Work out the finished part from the listing and answer in its coordinate system (mm). Face numbers are marked on the shaded views. Coordinates: 2 decimals unless noted, no trailing zeros. Loops run counter-clockwise (first coordinate to the right, second up) from the corner with the lowest first, then second, coordinate; pieces in that order, holes last. Notation, with made-up numbers: M -10.5,25 L 38.5,25 A22 cw 38.5,31 Z; hole C -15.5,34.25 d4. An arc over 180 degrees is marked long. Write each question's results on one line, items separated by ' | '.
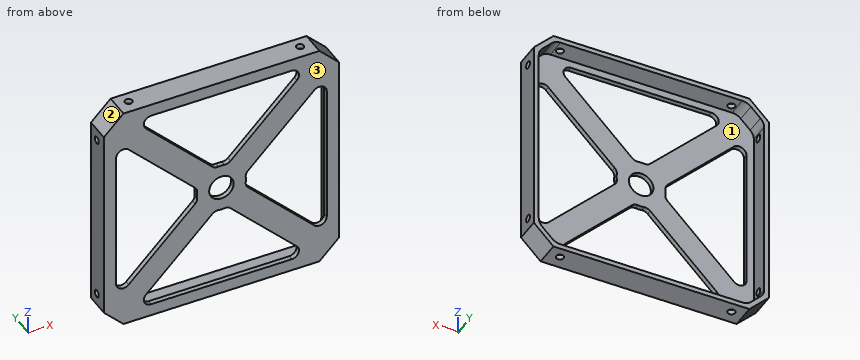
```python
from build123d import *

# Parameters (mm, degrees)
BOSS_EXTRUDE1_DEPTH = 10
SHELL1_T            = -2
SKETCH2_R           = 5
CUT_EXTRUDE1_DEPTH  = 11
FILLET1_R           = 3
SKETCH3_R           = 1.5
CUT_EXTRUDE2_DEPTH  = 97
SKETCH4_R           = 1.5
CUT_EXTRUDE3_DEPTH  = 97
FILLET2_R           = 5


with BuildPart() as part:
    # Sketch1 → Boss-Extrude1 (new body)
    with BuildSketch(Plane(origin=(0, 0, 0), x_dir=(1, 0, 0), z_dir=(0, 1, 0))):
        Polygon((0, 88), (0, 8), (8, 0), (88, 0), (96, 8), (96, 88), (88, 96), (8, 96), align=None)
    extrude(amount=BOSS_EXTRUDE1_DEPTH)

    # Shell1
    shell1_openings = [part.faces().sort_by_distance(p)[0] for p in [
        (48, 10, -48),
    ]]
    offset(amount=SHELL1_T, openings=shell1_openings, kind=Kind.INTERSECTION)

    # Sketch2 → Cut-Extrude1 (cut, through all)
    with BuildSketch(Plane(origin=(0, 0, 0), x_dir=(-1, 0, 0), z_dir=(0, -1, 0))):
        with BuildLine():
            Line((-45.411809549, 57.659258263), (-12.071067812, 91))
            Line((-12.071067812, 91), (-83.928932188, 91))
            Line((-83.928932188, 91), (-50.588190451, 57.659258263))
            ThreePointArc((-50.588190451, 57.659258263), (-48, 58), (-45.411809549, 57.659258263))
        make_face()
        with BuildLine():
            Line((-5, 83.928932188), (-38.340741737, 50.588190451))
            ThreePointArc((-38.340741737, 50.588190451), (-38.085551386, 49.305261922), (-38, 48))
            ThreePointArc((-38, 48), (-38.085551386, 46.694738078), (-38.340741737, 45.411809549))
            Line((-38.340741737, 45.411809549), (-5, 12.071067812))
            Line((-5, 12.071067812), (-5, 83.928932188))
        make_face()
        with BuildLine():
            Line((-12.071067812, 5), (-45.411809549, 38.340741737))
            ThreePointArc((-45.411809549, 38.340741737), (-48, 38), (-50.588190451, 38.340741737))
            Line((-50.588190451, 38.340741737), (-83.928932188, 5))
            Line((-83.928932188, 5), (-12.071067812, 5))
        make_face()
        with BuildLine():
            ThreePointArc((-57.659258263, 45.411809549), (-58, 48), (-57.659258263, 50.588190451))
            Line((-57.659258263, 50.588190451), (-91, 83.928932188))
            Line((-91, 83.928932188), (-91, 12.071067812))
            Line((-91, 12.071067812), (-57.659258263, 45.411809549))
        make_face()
        with Locations((-48, 48)):
            Circle(SKETCH2_R)
    extrude(amount=-CUT_EXTRUDE1_DEPTH, mode=Mode.SUBTRACT)

    # Fillet1
    fillet1_edges = [part.edges().sort_by_distance(p)[0] for p in [
        (50.588190451, 1, -38.340741737),
        (45.411809549, 1, -38.340741737),
        (12.071067812, 1, -5),
        (83.928932188, 1, -5),
        (38.340741737, 1, -45.411809549),
        (38.340741737, 1, -50.588190451),
        (5, 1, -83.928932188),
        (5, 1, -12.071067812),
        (57.659258263, 1, -50.588190451),
        (57.659258263, 1, -45.411809549),
        (91, 1, -12.071067812),
        (91, 1, -83.928932188),
        (45.411809549, 1, -57.659258263),
        (50.588190451, 1, -57.659258263),
        (83.928932188, 1, -91),
        (12.071067812, 1, -91),
    ]]
    fillet(fillet1_edges, radius=FILLET1_R)

    # Sketch3 → Cut-Extrude2 (cut, through all)
    with BuildSketch(Plane(origin=(96, 0, 0), x_dir=(0, 0, -1), z_dir=(1, 0, 0))):
        with Locations((83, 5.5)):
            Circle(SKETCH3_R)
        with Locations((13, 5.5)):
            Circle(SKETCH3_R)
    extrude(amount=-CUT_EXTRUDE2_DEPTH, mode=Mode.SUBTRACT)

    # Sketch4 → Cut-Extrude3 (cut, through all)
    with BuildSketch(Plane.XY):
        with Locations((83, 5.5)):
            Circle(SKETCH4_R)
        with Locations((13, 5.5)):
            Circle(SKETCH4_R)
    extrude(amount=-CUT_EXTRUDE3_DEPTH, mode=Mode.SUBTRACT)

    # Fillet2
    fillet2_edges = [part.edges().sort_by_distance(p)[0] for p in [
        (8.828427125, 6, -94),
        (2, 6, -87.171572875),
        (2, 6, -8.828427125),
        (8.828427125, 6, -2),
        (87.171572875, 6, -2),
        (94, 6, -8.828427125),
        (94, 6, -87.171572875),
        (87.171572875, 6, -94),
    ]]
    fillet(fillet2_edges, radius=FILLET2_R)


solid = part.part
```
1) For a pull along X with two mould halves and no side action, classify the marked faces 1, 2 and 3 as released by +X, released by -X, zero draft, split by the parting line, or undercut.
Check result:
face 1: undercut | face 2: released by -X | face 3: zero draft
2) Given pin 1 Ø6 at (x, y) = (62.5, 7) entering from +Z; pin 2 Ø4 at (x, z) = (51.5, -43.5) entering from +Y, each flat-ended and moving along its own axis, determine where each tip first touches the part or whether it passes through.
Check result:
pin 1: z = 0 | pin 2: y = 2
3) Find section B-B, the plane z = -13. Give the vertices of the cut face in (x, y).
Check result:
outline: M 0,0 L 20.07,0 L 20.07,2 L 2,2 L 2,4 L 0,4 Z; M 0,7 L 2,7 L 2,10 L 0,10 Z; M 75.93,0 L 96,0 L 96,4 L 94,4 L 94,2 L 75.93,2 Z; M 94,7 L 96,7 L 96,10 L 94,10 Z
4) Find section A-A, the plane x = 48. Give the vertices of the cut face in (y, z), and give its area (3 significant figures).
Check result:
outline: M 0,-96 L 10,-96 L 10,-94 L 2,-94 L 2,-91 L 0,-91 Z; M 0,-58 L 2,-58 L 2,-53 L 0,-53 Z; M 0,-43 L 2,-43 L 2,-38 L 0,-38 Z; M 0,-5 L 2,-5 L 2,-2 L 10,-2 L 10,0 L 0,0 Z | area: 72.0 mm^2
5) Straight lines are drawn through the part: probe 1 along Z at (x, y) = (48, 1.4); probe 2 along Z at (x, y) = (16, 2.5); probe 3 along X at (y, z) = (9.25, -20.5). For each, find the intervals that lie inside material, in ascending order. Write a range as [from, to].
Check result:
probe 1: [-96, -91], [-58, -53], [-43, -38], [-5, 0] | probe 2: [-96, -94], [-2, 0] | probe 3: [0, 2], [94, 96]
